Verification items for the finished model (mm, model axes). Face numbers are marked on the shaded views. A direction names the side the tool comes from. Round coordinates to 2 decimals unless told otherwise and drop trailing zeros. Write each loop counter-clockwise with the first axis right and the second up, starting at its lowest first coordinate (ties: lowest second). Pieces come first, ordered by that corner, then holes. Notation, with made-up numbers: M -21.5,75 L 23.5,75 A33 cw 23.5,104 Z; hole C 41.5,-36.75 d4. An arc over 180 degrees is marked long. One line per question, with ' | ' between items.
from build123d import *

# Parameters (mm, degrees)
F0_W     = 300
F0_H     = 400
F1_DEPTH = 10
F2_R     = 35
F3_DEPTH = 10
F4_R     = 70
F5_DEPTH = 10


with BuildPart() as f1:
    # F0 (on Top) → F1 (new body)
    with BuildSketch(Plane.XY):
        Rectangle(F0_W, F0_H)
    extrude(amount=F1_DEPTH)

    # F2 (on face) → F3 (join)
    with BuildSketch(Plane.XY.offset(10)):
        with Locations((-75, 125)):
            Circle(F2_R)
    extrude(amount=F3_DEPTH)

    # F4 (on face) → F5 (join)
    with BuildSketch(Plane.XY.offset(10)):
        Circle(F4_R)
    extrude(amount=F5_DEPTH)


solid = f1.part
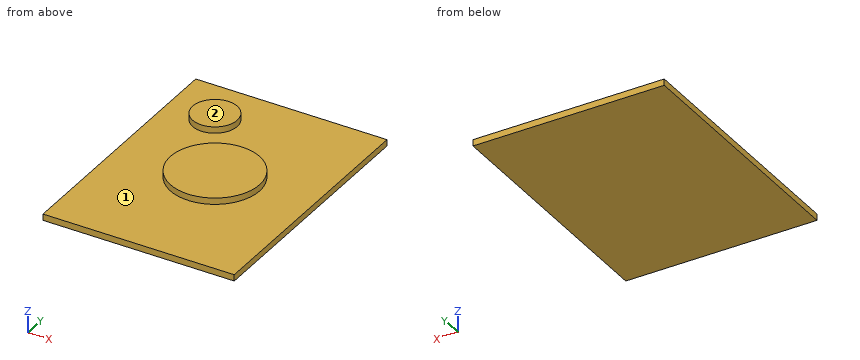
1. Go/stop test with a flat-tipped pin: P1, Ø1.5, axis at x = 23.5, y = -91.5, coming from the +Z side. Record where the tip stops, or that it passes through.
Results:
P1: stops at z = 10
2. Tool access check on the marked faces 1 and 2. Record the directions out of +Z, -Z, +X, -X, +Y, -Y that give a thin tool (end or side, any length) a straight path to the whole face; none if there is none.
Results:
face 1: +Z | face 2: +Z, +X, -X, +Y, -Y
3. Section check D-D, the plane x = 118. Record the cut outline in (y, z), then the cut area to 3 significant figures.
Results:
outline: M -200,0 L 200,0 L 200,10 L -200,10 Z | area: 4,000 mm2
4. Thickness scan on line 1 (Z direction, x = 79.5, y = 173); line 2 (Y direction, x = -63.5, z = 15); line 3 (Y direction, x = 31.5, z = 16.75). Record the ranges inside material, lowest first.
Results:
line 1: z = 0 to 10 | line 2: y = -29.46 to 29.46, 91.94 to 158.06 | line 3: y = -62.51 to 62.51
5. Section check B-B, the plane y = 125. Record the cut outline in (x, z), then the cut area to 3 significant figures.
Results:
outline: M -150,0 L 150,0 L 150,10 L -40,10 L -40,20 L -110,20 L -110,10 L -150,10 Z | area: 3,700 mm2
6. Section check A-A, the plane x = -75. Record the cut outline in (y, z), then the cut area to 3 significant figures.
Results:
outline: M -200,0 L 200,0 L 200,10 L 160,10 L 160,20 L 90,20 L 90,10 L -200,10 Z | area: 4,700 mm2
7. Section check C-C, the plane z = 14. Record the cut outline in (x, y).
Results:
outline: C -75,125 d70; C 0,0 d140
